Design review of the part built by this model. Coordinates are the model's own, in mm. A direction names the side the tool comes from. Give positions to 0.01 mm unless a question says otherwise; leave off trailing zeros. Write each loop counter-clockwise with the first axis right and the second up, starting at its lowest first coordinate (ties: lowest second). Pieces come first, ordered by that corner, then holes. Notation, with made-up numbers: M 36,83.5 L 67,83.5 A10 ccw 67,94.5 Z; hole C -11,14 d10. An arc over 180 degrees is marked long. Answer in a Markdown table with one row per item.
```python
from build123d import *

# Parameters (mm, degrees)
F0_R     = 45
F1_DEPTH = 25.4
F2_R     = 42.5
F3_DEPTH = 23.4
F4_R     = 7.25
F5_DEPTH = 25


with BuildPart() as f1:
    # F0 (on Top) → F1 (new body)
    with BuildSketch(Plane.XY):
        Circle(F0_R)
    extrude(amount=F1_DEPTH)

    # F2 (on face) → F3 (cut, through all)
    with BuildSketch(Plane.XY.offset(25.4)):
        Circle(F2_R)
    extrude(amount=-F3_DEPTH, mode=Mode.SUBTRACT)

    # F4 (on face) → F5 (cut)
    with BuildSketch(Plane.XY.offset(2)):
        Circle(F4_R)
    extrude(amount=-F5_DEPTH, mode=Mode.SUBTRACT)


solid = f1.part
```
1) Insertion check: P1, Ø8, axis at y = -21, z = 5, coming from the +X side; P2, Ø8.5, axis at x = 0, y = 0, coming from the +Z side; P3, Ø8, axis at x = 14.5, z = 9.5, coming from the +Y side; P4, Ø3, axis at x = -20, y = -8, coming from the +Z side. Each pin has a flat end and moves straight along its axis. Give the tip position at first contact, or say it passes through.
Geometry says:
| item | result |
|---|---|
| P1 | x = 41.67 |
| P2 | through |
| P3 | y = 43.76 |
| P4 | z = 2 |
2) Add section A-A (y = 0). Write out the cut boundary in (x, z).
Geometry says:
| item | result |
|---|---|
| outline | M -45,0 L -7.25,0 L -7.25,2 L -42.5,2 L -42.5,25.4 L -45,25.4 Z; M 7.25,0 L 45,0 L 45,25.4 L 42.5,25.4 L 42.5,2 L 7.25,2 Z |
3) The part is to be moulded in two halves that separate along X. For faces 1 (the face through (-1, -9, 0)), 2 (the face through (20.765, -39.923, 12.522)), 3 (the face through (-1, -9, 2)), say which applies: released by +X, released by -X, zero draft, split by the parting line, or undercut.
Geometry says:
| item | result |
|---|---|
| face 1 | zero draft |
| face 2 | split by the parting line |
| face 3 | undercut |
4) For faces 4 (the face through (3.35, -6.43, 1.01)), 5 (the face through (-33.727, -25.861, 13.864)), list the 3-axis set-ups (+Z, -Z, +X, -X, +Y, -Y) from which the entire face can be reached by the end or side of a thin tool; tool diameter is ignored.
Geometry says:
| item | result |
|---|---|
| face 4 | +Z, -Z |
| face 5 | +Z |
5) Add section D-D (x = 30). Write out the cut boundary in (y, z).
Geometry says:
| item | result |
|---|---|
| outline | M -33.54,0 L 33.54,0 L 33.54,25.4 L 30.1,25.4 L 30.1,2 L -30.1,2 L -30.1,25.4 L -33.54,25.4 Z |
6) To check wall thickness, follow probe 1 along Y at (x, z) = (0, 18); probe 2 along Z at (x, y) = (32.5, 10.5); probe 3 along Y at (x, z) = (0, 1). State the ranges of each line that lie inside material, in increasing order. Write a range as [from, to].
Geometry says:
| item | result |
|---|---|
| probe 1 | [-45, -42.5], [42.5, 45] |
| probe 2 | [0, 2] |
| probe 3 | [-45, -7.25], [7.25, 45] |
7) Add section C-C (z = 6.5). Write out the cut boundary in (x, y).
Geometry says:
| item | result |
|---|---|
| outline | C 0,0 d90; hole C 0,0 d85 |
